from build123d import *

# Parameters (mm, degrees)
BOSS_EXTRUDE1_DEPTH = 10
SKETCH2_R           = 2.5
CUT_EXTRUDE1_DEPTH  = 31.22831719


with BuildPart() as part:
    # Sketch1 → Boss-Extrude1 (new body)
    with BuildSketch(Plane.XY):
        with BuildLine():
            Line((-18.283811633, 4.93818979), (-14.865726836, 4.93818979))
            ThreePointArc((-14.865726836, 4.93818979), (-14.726980342, 4.84519339), (-14.760272841, 4.681515262))
            Line((-14.760272841, 4.681515262), (-18.546923839, 0.93818979))
            Line((-18.546923839, 0.93818979), (-24.41329202, 0.93818979))
            Line((-24.41329202, 0.93818979), (-28.199943018, 4.681515262))
            ThreePointArc((-28.199943018, 4.681515262), (-28.233235517, 4.84519339), (-28.094489023, 4.93818979))
            Line((-28.094489023, 4.93818979), (-24.676404226, 4.93818979))
            Line((-24.676404226, 4.93818979), (-18.283811633, 4.93818979))
        make_face()
    extrude(amount=BOSS_EXTRUDE1_DEPTH)

    # Sketch2 → Cut-Extrude1 (cut, through all)
    with BuildSketch(Plane(origin=(0, 4.93818979, 0), x_dir=(1, 0, 0), z_dir=(0, 1, 0))):
        with Locations(Location((-21.480107929, -5, 0), (0, 0, 180))):
            Circle(SKETCH2_R)
    extrude(amount=-CUT_EXTRUDE1_DEPTH, mode=Mode.SUBTRACT)


solid = part.part
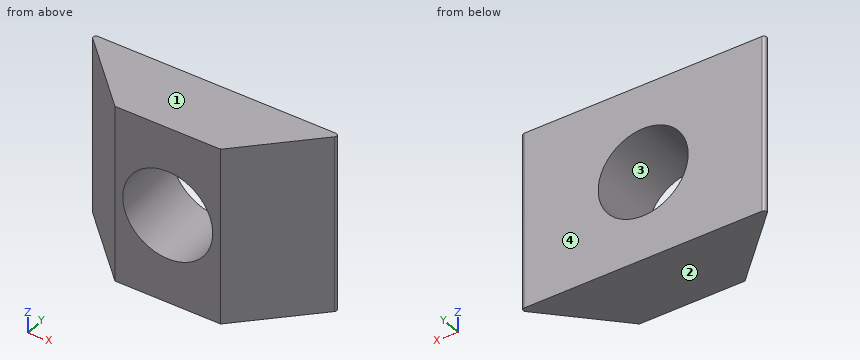
Design review of the part built by this model. Coordinates are the model's own, in mm. Face numbers are marked on the shaded views. Round coordinates to 2 decimals unless told otherwise and drop trailing zeros. Write each loop counter-clockwise with the first axis right and the second up, starting at its lowest first coordinate (ties: lowest second). Pieces come first, ordered by that corner, then holes. Notation, with made-up numbers: (19.5, -39.5) - (37.5, -39.5) arc R17 cw to (37.5, -30.5) - close; hole circle Ø5 at (30.5, 71.25). An arc over 180 degrees is marked (long way). Use a Markdown table: item, result. Add a question column.
1. We need section D-D (y = 2.15). State the section outline as (x, z) points, then the cut area to 3 significant figures.
2. Mouldability with a two-part tool opening along Z and no side actions: class the marked faces 1, 2, 3 and 4 as +Z half, -Z half, draft (parallel to the pull), parting line (faces both ways), or undercut.
3. Wall thickness on probe 1 along Z at (x, y) = (-21.5, 4.7); probe 2 along Z at (x, y) = (-20.75, 3.85); probe 3 along X at (y, z) = (4.4, 5.5): over which ranges is each line inside the solid? List them lowest first.
4. We need section B-B (x = -21). State the section outline as (y, z) points, then the cut area to 3 significant figures.
5. We need section C-C (z = 2.25). State the section outline as (x, y) points, then the cut area to 3 significant figures.
6. We need section A-A (z = 5). State the section outline as (x, y) points.
Output:
| question | item | result |
|---|---|---|
| 1 | outline | (-25.64, 0) - (-17.32, 0) - (-17.32, 10) - (-25.64, 10) - close; hole circle Ø5 at (-21.48, 5) |
| 1 | area | 63.5 mm2 |
| 2 | face 1 | +Z half |
| 2 | face 2 | -Z half |
| 2 | face 3 | undercut |
| 2 | face 4 | draft |
| 3 | probe 1 | z = 0 to 2.5, 7.5 to 10 |
| 3 | probe 2 | z = 0 to 2.61, 7.39 to 10 |
| 3 | probe 3 | x = -27.92 to -23.93, -19.03 to -15.05 |
| 4 | outline | (0.94, 0) - (4.94, 0) - (4.94, 2.55) - (0.94, 2.55) - close; (0.94, 7.45) - (4.94, 7.45) - (4.94, 10) - (0.94, 10) - close |
| 4 | area | 20.4 mm2 |
| 5 | outline | (-28.2, 4.68) - (-24.41, 0.94) - (-18.55, 0.94) - (-14.76, 4.68) arc R0.15 ccw to (-14.87, 4.94) - (-28.09, 4.94) arc R0.15 ccw to start |
| 5 | area | 39.6 mm2 |
| 6 | outline | (-28.2, 4.68) - (-24.41, 0.94) - (-23.98, 0.94) - (-23.98, 4.94) - (-28.09, 4.94) arc R0.15 ccw to start; (-18.98, 0.94) - (-18.55, 0.94) - (-14.76, 4.68) arc R0.15 ccw to (-14.87, 4.94) - (-18.98, 4.94) - close |
